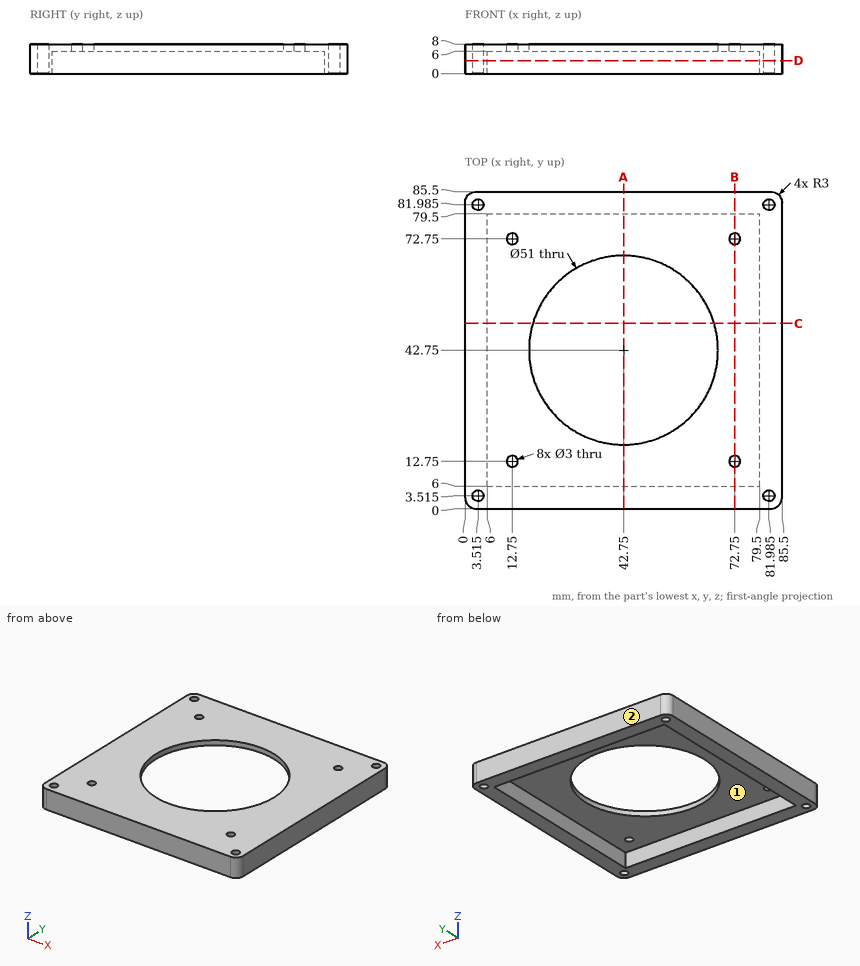
Check sheet for the drawn part. Datum: minimum x, y, z corner. Units: mm. A direction names the side the tool comes from. Give positions to 0.01 mm unless a question says otherwise; leave off trailing zeros. Loops run counter-clockwise (first coordinate to the right, second up) from the corner with the lowest first, then second, coordinate; pieces in that order, holes last.
1) Sectioned sample at B-B, the plane x = 72.75. Enter the section's corners in (y, z), then the cut area to 3 significant figures.
2) Thickness scan on line 1 along Y through (x, z) = (72.75, 6.8); line 2 along X through (y, z) = (15, 1.5). Record the ranges inside material, lowest first.
3) Sectioned sample at C-C, the plane y = 50. Enter the section's corners in (x, z).
4) Sectioned sample at A-A, the plane x = 42.75. Enter the section's corners in (y, z), then the cut area to 3 significant figures.
5) Depth check by flat-ended pin: pin 1 Ø4 at (x, y) = (12.75, 72.75) entering from -Z. Enter the tip coordinate at first touch or a pass-through.
6) Set-up check for the marked faces 1 and 2: record each of +Z, -Z, +X, -X, +Y, -Y from which the full face is reachable in a straight line by a thin tool's end or side.
7) Sectioned sample at D-D, the plane z = 3.5. Enter the section's corners in (x, y) (1 decimal).
Answers:
1. outline: (0, 0) - (6, 0) - (6, 6) - (11.25, 6) - (11.25, 8) - (0, 8) - close; (14.25, 6) - (71.25, 6) - (71.25, 8) - (14.25, 8) - close; (74.25, 6) - (79.5, 6) - (79.5, 0) - (85.5, 0) - (85.5, 8) - (74.25, 8) - close
1. area: 231 mm2
2. line 1: y = 0 to 11.25, 14.25 to 71.25, 74.25 to 85.5
2. line 2: x = 0 to 6, 79.5 to 85.5
3. outline: (0, 0) - (6, 0) - (6, 6) - (18.3, 6) - (18.3, 8) - (0, 8) - close; (67.2, 6) - (79.5, 6) - (79.5, 0) - (85.5, 0) - (85.5, 8) - (67.2, 8) - close
4. outline: (0, 0) - (6, 0) - (6, 6) - (17.25, 6) - (17.25, 8) - (0, 8) - close; (68.25, 6) - (79.5, 6) - (79.5, 0) - (85.5, 0) - (85.5, 8) - (68.25, 8) - close
4. area: 141 mm2
5. pin 1: stops at z = 6
6. face 1: -Z
6. face 2: +Z, -Z, +X, -X, +Y
7. outline: (0, 3) arc R3 ccw to (3, 0) - (82.5, 0) arc R3 ccw to (85.5, 3) - (85.5, 82.5) arc R3 ccw to (82.5, 85.5) - (3, 85.5) arc R3 ccw to (0, 82.5) - close; hole circle Ø3 at (3.5, 3.5); hole circle Ø3 at (3.5, 82); hole (6, 6) - (79.5, 6) - (79.5, 79.5) - (6, 79.5) - close; hole circle Ø3 at (82, 3.5); hole circle Ø3 at (82, 82)
